from build123d import *

# Parameters (mm, degrees)
F0_W             = 20
F0_H             = 20
F1_DEPTH         = 433
F2_R             = 2.1
F3_DEPTH         = 433.001
F4_R             = 1
F6_DEPTH         = 433.001
F6_COPIES3_COUNT = 2
F6_COPIES3_ANGLE = 90
F6_COPIES4_COUNT = 2
F6_COPIES4_ANGLE = 270
F6_COPIES6_COUNT = 2
F9_W             = 16.4
F9_H             = 6.8613203436
F10_DEPTH        = 433.001
F12_DEPTH        = 433


# Not quite as in the source:
# - a pattern or mirror of a feature is missing from the dataset's text; its kind, count and spacing are read off the source's solid


with BuildPart() as f1:
    # F0 (on Front) → F1 (new body)
    with BuildSketch(Plane.XZ):
        Rectangle(F0_W, F0_H)
    extrude(amount=F1_DEPTH)

    # F2 (on face) → F3 (cut, through all)
    with BuildSketch(Plane.XZ.offset(433)):
        Circle(F2_R)
    extrude(amount=-F3_DEPTH, mode=Mode.SUBTRACT)

    # F4
    f4_edges = [f1.edges().sort_by_distance(p)[0] for p in [
        (-10, -216.5, 10),
        (10, -216.5, 10),
    ]]
    fillet(f4_edges, radius=F4_R)

    # F5 (on face) → F6 (cut, through all)
    with BuildSketch(Plane.XZ.offset(433)):
        Polygon((0, 3.9006601718), (0, 10), (-2.84, 10), (-4.64, 10), (-2.84, 8.2), (-5.4993398282, 8.2), (-5.4993398282, 6.56), (-2.84, 3.9006601718), align=None)
        Polygon((-6.5693398282, 8.2), (-8.2, 8.2), (-7.0953059148, 7.0953059148), (-6.5693398282, 7.6212720014), align=None)
    f6 = extrude(amount=-F6_DEPTH, mode=Mode.SUBTRACT)

    # F6_copies: F6 across plane
    add(f6.mirror(Plane(origin=(0, 0, 0), x_dir=(-0.7071067812, 0, -0.7071067812), z_dir=(0.7071067812, 0, -0.7071067812))), mode=Mode.SUBTRACT)

    # F6_copies1: F6 across plane
    add(f6.mirror(Plane(origin=(0, 0, 0), x_dir=(0.7071067812, 0, -0.7071067812), z_dir=(-0.7071067812, 0, -0.7071067812))), mode=Mode.SUBTRACT)

    # F6_copies2: F6 across plane
    add(f6.mirror(Plane(origin=(0, 0, 0), x_dir=(0, 0, 1), z_dir=(1, 0, 0))), mode=Mode.SUBTRACT)

    # F6_copies3: F6 ×2 about axis
    f6_copies3_axis = Axis((0, 0, 0), (0, 1, 0))
    for i in range(1, F6_COPIES3_COUNT):
        add(f6.rotate(f6_copies3_axis, i * F6_COPIES3_ANGLE / (F6_COPIES3_COUNT - 1)), mode=Mode.SUBTRACT)

    # F6_copies4: F6 ×2 about axis
    f6_copies4_axis = Axis((0, 0, 0), (0, 1, 0))
    for i in range(1, F6_COPIES4_COUNT):
        add(f6.rotate(f6_copies4_axis, i * F6_COPIES4_ANGLE / (F6_COPIES4_COUNT - 1)), mode=Mode.SUBTRACT)

    # F6_copies5: F6 across plane
    add(f6.mirror(Plane(origin=(0, 0, 0), x_dir=(-1, 0, 0), z_dir=(0, 0, -1))), mode=Mode.SUBTRACT)

    # F6_copies6: F6 ×2 about axis
    f6_copies6_axis = Axis((0, 0, 0), (0, 1, 0))
    for i in range(1, F6_COPIES6_COUNT):
        add(f6.rotate(f6_copies6_axis, i * 360 / F6_COPIES6_COUNT), mode=Mode.SUBTRACT)

    # F8: F1 across face


with BuildPart() as f1_1:
    add(f1.part)
    add(f1.part.mirror(Plane(origin=(-7.32, -216.5, -10), x_dir=(1, 0, 0), z_dir=(0, 0, -1))))

    # F9 (on face) → F10 (cut, through all)
    with BuildSketch(Plane.XZ.offset(433)):
        with Locations((0, -10)):
            Rectangle(F9_W, F9_H)
    extrude(amount=-F10_DEPTH, mode=Mode.SUBTRACT)

    # F11 (on face) → F12 (join, through all)
    with BuildSketch(Plane.XZ.offset(433)):
        with BuildLine():
            ThreePointArc((-9, -10), (-9.7071067812, -9.7071067812), (-10, -9))
            Line((-10, -9), (-10, -11))
            ThreePointArc((-10, -11), (-9.7071067812, -10.2928932188), (-9, -10))
        make_face()
        with BuildLine():
            ThreePointArc((10, -9), (9.7071067812, -9.7071067812), (9, -10))
            ThreePointArc((9, -10), (9.7071067812, -10.2928932188), (10, -11))
            Line((10, -11), (10, -9))
        make_face()
        Polygon((5.9386796564, -6.9993398282), (8.2, -6.9993398282), (8.2, -6.5693398282), (5.5086796564, -6.5693398282), align=None)
        Polygon((-8.2, -6.5693398282), (-8.2, -6.9993398282), (-5.9386796564, -6.9993398282), (-5.5086796564, -6.5693398282), align=None)
    extrude(amount=-F12_DEPTH)


solid = f1_1.part
Here's how the part is built. I have some questions about the finished solid (model axes, mm). Coordinates: 2 decimals unless noted, no trailing zeros.
1) If I drill on line 1 (Z direction, x = 0, y = -312.5); line 2 (X direction, y = -118, z = -8.5); line 3 (Z direction, x = 7.25, y = -265), over which ranges is the centre line in solid material (lowest first)?
Filled in:
line 1: z = -23.9 to -22.1, -17.9 to -16.1, -3.9 to -2.1, 2.1 to 3.9
line 2: x = -10 to -8.2, 8.2 to 10
line 3: z = -30 to -28.2, -26.94 to -25.5, -14.5 to -13.43, -7 to -5.5, 5.5 to 6.94, 8.2 to 10
2) I'm going to push flat-ended pins straight in: pin 1 (2 mm diameter, centred on y = -245.5, z = -16.5, fed in from -X); pin 2 (3 mm diameter, centred on x = 4.5, y = -236.5, fed in from +Z); pin 3 (1.7 mm diameter, centred on y = -142.5, z = 1.5, fed in from -X); pin 4 (1 mm diameter, centred on x = 0, y = -285, fed in from +Z). Where does each tip first touch, or does it pass through?
Filled in:
pin 1: stops at x = -9.86
pin 2: stops at z = 10
pin 3: stops at x = -3.9
pin 4: stops at z = 3.9
3) If we section it at A-A (y = -388): Count the separate pieces of the cut face and the enclosed holes in it, plus the area to 3 significant figures.
Filled in:
separate pieces: 1
enclosed holes: 7
area: 286 mm2
